```python
from build123d import *

# Parameters (mm, degrees)
BOSS_EXTRUDE1_DEPTH = 25.4
SKETCH2_R           = 2.25
CUT_EXTRUDE1_DEPTH  = 88.290380725
FILLET1_R           = 2


with BuildPart() as part:
    # Sketch1 → Boss-Extrude1 (new body)
    with BuildSketch(Plane.XY):
        with BuildLine():
            Line((-12.3952, 40.3748), (-12.3952, 0))
            Line((-12.3952, 0), (-12.3952, -22.2504))
            Line((-12.3952, -22.2504), (-13.0952, -22.2504))
            ThreePointArc((-13.0952, -22.2504), (-21.580481374, -18.735681374), (-25.0952, -10.2504))
            Line((-25.0952, -10.2504), (-25.0952, 30.1244))
            Line((-25.0952, 30.1244), (-25.0952, 52.3748))
            Line((-25.0952, 52.3748), (-24.3952, 52.3748))
            ThreePointArc((-24.3952, 52.3748), (-15.909918626, 48.860081374), (-12.3952, 40.3748))
        make_face()
        with BuildLine():
            ThreePointArc((-37.4904, 50.3748), (-36.904613562, 51.789013562), (-35.4904, 52.3748))
            Line((-35.4904, 52.3748), (-25.0952, 52.3748))
            Line((-25.0952, 52.3748), (-25.0952, 30.1244))
            Line((-25.0952, 30.1244), (-35.4904, 30.1244))
            ThreePointArc((-35.4904, 30.1244), (-36.904613562, 30.710186438), (-37.4904, 32.1244))
            Line((-37.4904, 32.1244), (-37.4904, 50.3748))
        make_face()
        with BuildLine():
            ThreePointArc((0, -20.2504), (-0.585786438, -21.664613562), (-2, -22.2504))
            Line((-2, -22.2504), (-12.3952, -22.2504))
            Line((-12.3952, -22.2504), (-12.3952, 0))
            Line((-12.3952, 0), (-2, 0))
            ThreePointArc((-2, 0), (-0.585786438, -0.585786438), (0, -2))
            Line((0, -2), (0, -20.2504))
        make_face()
    extrude(amount=BOSS_EXTRUDE1_DEPTH)

    # Sketch2 → Cut-Extrude1 (cut, through all)
    with BuildSketch(Plane(origin=(0, 52.3748, 0), x_dir=(1, 0, 0), z_dir=(0, 1, 0))):
        with Locations(Location((-31.4452, -6.35, 0), (0, 0, 270))):
            Circle(SKETCH2_R)
        with Locations(Location((-31.4452, -19.05, 0), (0, 0, 270))):
            Circle(SKETCH2_R)
        with Locations(Location((-6.0452, -6.35, 0), (0, 0, 270))):
            Circle(SKETCH2_R)
        with Locations(Location((-6.0452, -19.05, 0), (0, 0, 270))):
            Circle(SKETCH2_R)
    extrude(amount=-CUT_EXTRUDE1_DEPTH, mode=Mode.SUBTRACT)

    # Fillet1
    fillet1_edges = [part.edges().sort_by_distance(p)[0] for p in [
        (-15.909918626, 48.860081374, 25.4),
        (-29.9428, 52.3748, 25.4),
        (-7.1976, 0, 0),
        (-0.585786438, -0.585786438, 0),
        (0, -11.1252, 0),
        (-0.585786438, -21.664613562, 0),
        (-7.5476, -22.2504, 0),
        (-21.580481374, -18.735681374, 0),
        (-25.0952, 9.937, 0),
        (-30.2928, 30.1244, 0),
        (-36.904613562, 30.710186438, 0),
        (-37.4904, 41.2496, 0),
        (-36.904613562, 51.789013562, 0),
        (-29.9428, 52.3748, 0),
        (-15.909918626, 48.860081374, 0),
        (-36.904613562, 51.789013562, 25.4),
        (-12.3952, 20.1874, 0),
        (-37.4904, 41.2496, 25.4),
        (-36.904613562, 30.710186438, 25.4),
        (-30.2928, 30.1244, 25.4),
        (-25.0952, 9.937, 25.4),
        (-21.580481374, -18.735681374, 25.4),
        (-12.3952, 20.1874, 25.4),
        (-7.5476, -22.2504, 25.4),
        (-0.585786438, -21.664613562, 25.4),
        (0, -11.1252, 25.4),
        (-0.585786438, -0.585786438, 25.4),
        (-7.1976, 0, 25.4),
    ]]
    fillet(fillet1_edges, radius=FILLET1_R)


solid = part.part
```
Input: part model. Units: mm. Frame: model coordinates. A direction names the side the tool comes from. Give positions to 0.01 mm unless a question says otherwise; leave off trailing zeros. Order: outer loops, then holes, each group sorted by start corner. A loop starts at its lowest first (then second) coordinate and runs counter-clockwise, first axis right, second up.
1. Cut plane A-A (x = -9.5). Return loops of the section in (y, z).
Computed:
outline: (-22.25, 2) arc R2 ccw to (-20.25, 0) - (-2, 0) arc R2 ccw to (0, 2) - (0, 23.4) arc R2 ccw to (-2, 25.4) - (-20.25, 25.4) arc R2 ccw to (-22.25, 23.4) - close
2. Line query: probe 1 along X at (y, z) = (-9.75, 19.05); probe 2 along X at (y, z) = (37.5, 6.35); probe 3 along Y at (x, z) = (-34.5, 4.75). Output: solid intervals per line, ascending.
Computed:
probe 1: x = -25.1 to -8.3, -3.8 to 0
probe 2: x = -37.49 to -33.7, -29.2 to -12.4
probe 3: y = 30.12 to 52.37
3. Pin query (flat end, axial travel): pin 1 Ø1.5 at (x, z) = (-7, 19.5) entering from +Y; pin 2 Ø2 at (x, z) = (-14.5, 20) entering from +Y; pin 3 Ø6.5 at (y, z) = (26, 10.5) entering from +X; pin 4 Ø3 at (x, z) = (-30.5, 12.5) entering from -Y. Return the tip coordinate at first contact, or that it passes through.
Computed:
pin 1: passes through
pin 2: stops at y = 48.43
pin 3: stops at x = -12.4
pin 4: stops at y = 30.12
4. Draft query along X for faces 5 (the face through (-29.214, 41.405, 6.057)), 6 (the face through (-5.946, -10.969, 16.802)), 7 (the face through (-29.865, 51.804, 24.799)), 8 (the face through (-0.57, -11.25, 0.6)). Return one class per face: released by +X, released by -X, zero draft, split by the parting line, or undercut.
Computed:
face 5: undercut
face 6: undercut
face 7: zero draft
face 8: released by +X
5. Cut plane C-C (y = 19.5). Return loops of the section in (x, z), and give its area (3 significant figures).
Computed:
outline: (-25.1, 2) arc R2 ccw to (-23.1, 0) - (-14.4, 0) arc R2 ccw to (-12.4, 2) - (-12.4, 23.4) arc R2 ccw to (-14.4, 25.4) - (-23.1, 25.4) arc R2 ccw to (-25.1, 23.4) - close
area: 319 mm2
6. Cut plane D-D (z = 12). Return loops of the section in (x, y).
Computed:
outline: (-37.49, 32.12) arc R2 ccw to (-35.49, 30.12) - (-25.1, 30.12) - (-25.1, -10.25) arc R12 ccw to (-13.1, -22.25) - (-2, -22.25) arc R2 ccw to (0, -20.25) - (0, -2) arc R2 ccw to (-2, 0) - (-12.4, 0) - (-12.4, 40.37) arc R12 ccw to (-24.4, 52.37) - (-35.49, 52.37) arc R2 ccw to (-37.49, 50.37) - close
7. Set-up query: faces 1 (the face through (-19, 16, 25.4)), 2 (the face through (-29.38, 30.726, 0.57)), 3 (the face through (-25.095, 10, 13)), 4 (the face through (-8.11, -0.6, 24.83)). Return all of +Z, -Z, +X, -X, +Y, -Y with unobstructed straight access to the full face (end or side cutting, diameter ignored); none if empty.
Computed:
face 1: +Z, +X, -X, +Y, -Y
face 2: -Z, -X, -Y
face 3: +Z, -Z, -X, -Y
face 4: +Z, +X, +Y
8. Cut plane B-B (z = 19.05). Return loops of the section in (x, y).
Computed:
outline: (-37.49, 32.12) arc R2 ccw to (-35.49, 30.12) - (-33.7, 30.12) - (-33.7, 52.37) - (-35.49, 52.37) arc R2 ccw to (-37.49, 50.37) - close; (-29.2, 30.12) - (-25.1, 30.12) - (-25.1, -10.25) arc R12 ccw to (-13.1, -22.25) - (-8.3, -22.25) - (-8.3, 0) - (-12.4, 0) - (-12.4, 40.37) arc R12 ccw to (-24.4, 52.37) - (-29.2, 52.37) - close; (-3.8, -22.25) - (-2, -22.25) arc R2 ccw to (0, -20.25) - (0, -2) arc R2 ccw to (-2, 0) - (-3.8, 0) - close
